Check sheet for the modelled part. Datum: model origin and axes. Units: mm. Face numbers are marked on the shaded views. A direction names the side the tool comes from. Coordinates: 2 decimals unless noted, no trailing zeros. Write each loop counter-clockwise with the first axis right and the second up, starting at its lowest first coordinate (ties: lowest second). Pieces come first, ordered by that corner, then holes. Notation, with made-up numbers: (-13, -35) -> (39, -35) arc R15 cw to (39, -14) -> close; hole circle Ø11 at (66.5, 21.5). An arc over 180 degrees is marked (long way). Put each result on its own line as item: value.
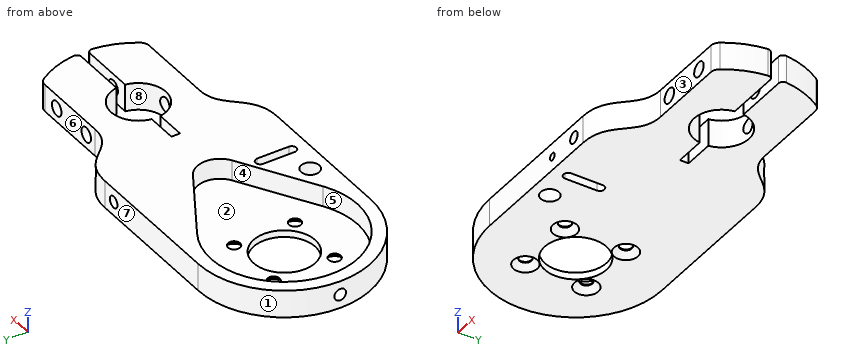
Autodesk Inventor part; units mm, degrees
ref_plane "Work Plane2" through (-108.2066, 0, 0) normal (1, 0, 0) x (0, 1, 0)
ref_plane "XZ Plane" through (0, 0, 0) normal (0, 1, 0) x (-1, 0, 0)
ref_plane "XY Plane" through (0, 0, 0) normal (0, 0, 1) x (1, 0, 0)
sketch "Sketch1" plane through (0, 0, 0) normal (0, 0, 1) x (1, 0, 0)
  circle A0 centre (-78.2066, 0) radius 10.75
  arc A1 (-78.2066, 30) -> (-78.2066, -30) centre (-78.2066, 0) ccw
  line L0 (-78.2066, 30) -> (-28.164, 30)
  line L1 (-28.164, -30) -> (-78.2066, -30)
  circle A2 centre (-88.8132, 10.6066) radius 2.1
  circle A3 centre (-67.6, -10.6066) radius 2.1
  circle A4 centre (-88.8132, -10.6066) radius 2.1
  circle A5 centre (-67.6, 10.6066) radius 2.1
  line L2 (-88.8132, 10.6066) -> (-67.6, -10.6066) construction
  line L3 (-67.6, 10.6066) -> (-88.8132, -10.6066) construction
  line L4 (-67.6, 10.6066) -> (-88.8132, 10.6066) construction
  line L5 (-67.6, 10.6066) -> (-67.6, -10.6066) construction
  line L6 (-135.9764, 0) -> (58.4124, 0)
  line L7 (9.4315, 1.5) -> (28.2442, 1.5)
  line L8 (28.2442, -1.5) -> (9.4315, -1.5)
  line L9 (-9.4315, 1.5) -> (-29.9625, 1.5)
  line L10 (-9.4315, -1.5) -> (-29.9625, -1.5)
  line L11 (-20, -1.5) -> (-20, 1.5)
  line L12 (9.55, -26.0565) -> (9.55, -21.3339)
  line L13 (12.725, -18.1589) -> (22.25, -18.1589)
  arc A6 (12.725, -18.1589) -> (9.55, -21.3339) centre (12.725, -21.3339) ccw
  arc A7 (7.1295, 29.1405) -> (0, 30) centre (0, 0) ccw
  arc A8 (9.4315, 1.5) -> (-9.4315, 1.5) centre (0, 0) ccw
  arc A9 (-9.4315, -1.5) -> (9.4315, -1.5) centre (0, 0) ccw
  arc A10 (24.8835, -16.7574) -> (29.8223, -3.26) centre (0, 0) ccw
  arc A11 (22.25, -18.1589) -> (24.8835, -16.7574) centre (22.25, -14.9839) ccw
  arc A12 (7.1295, -29.1405) -> (9.55, -26.0565) centre (6.375, -26.0565) ccw
  line L14 (9.55, 26.0565) -> (9.55, 21.3339)
  line L15 (12.725, 18.1589) -> (22.25, 18.1589)
  arc A13 (9.55, 21.3339) -> (12.725, 18.1589) centre (12.725, 21.3339) ccw
  arc A14 (29.8223, 3.26) -> (24.8835, 16.7574) centre (0, 0) ccw
  arc A15 (24.8835, 16.7574) -> (22.25, 18.1589) centre (22.25, 14.9839) ccw
  arc A16 (9.55, 26.0565) -> (7.1295, 29.1405) centre (6.375, 26.0565) ccw
  arc A17 (0, -30) -> (7.1295, -29.1405) centre (0, 0) ccw
  arc A18 (0, 30) -> (0, -30) centre (0, 0) ccw construction
  line L16 (-28.164, -30) -> (-14.7272, -30) construction
  line L17 (-14.7272, -30) -> (-16.1546, -18.1589) construction
  line L18 (-16.1546, -18.1589) -> (-4.7625, -18.1589) construction
  spline S0 degree 3 poles (-28.164, -30) (-14.7272, -30) (-16.1546, -18.1589) (-4.7625, -18.1589) knots 1 1 1 1 2 2 2 2
  arc A19 (28.2442, 1.5) -> (29.8223, 3.26) centre (28.2442, 3.0875) ccw
  arc A20 (29.8223, -3.26) -> (28.2442, -1.5) centre (28.2442, -3.0875) ccw
  line L19 (12.725, -18.1589) -> (-4.7625, -18.1589)
  line L20 (-28.164, 30) -> (-14.7272, 30) construction
  line L21 (-14.7272, 30) -> (-16.1546, 18.1589) construction
  line L22 (-16.1546, 18.1589) -> (-4.7625, 18.1589) construction
  spline S1 degree 3 poles (-28.164, 30) (-14.7272, 30) (-16.1546, 18.1589) (-4.7625, 18.1589) knots 1 1 1 1 2 2 2 2
  line L23 (12.725, 18.1589) -> (-4.7625, 18.1589)
  point P0 (-78.2066, 0)
  point P1 (9.55, -28.4394)
  point P2 (9.55, -18.1589)
  point P3 (23.88, -18.1589)
  point P4 (23.88, -18.1589)
  point P5 (29.9625, -1.5)
  point P6 (9.55, 28.4394)
  point P7 (9.55, 18.1589)
  point P8 (23.88, 18.1589)
  point P9 (23.88, 18.1589)
  point P10 (29.9625, 1.5)
  dimension "d2" = 21.5
  dimension "d3" = 78.2066
  dimension "d4" = 60
  dimension "d5" = 4.2
  dimension "d6" = 4.2
  dimension "d7" = 4.2
  dimension "d8" = 4.2
  dimension "d9" = 30
  dimension "d13" = 3
  dimension "d20" = 3
  dimension "d21" = 1.5
  dimension "d22" = 20
  dimension "d34" = 3.175
  dimension "d35" = 30
  dimension "d38" = 9.55
  dimension "d39" = 9.55
  dimension "d41" = 30
  dimension "d43" = 3.175
  dimension "d44" = 9.525
  dimension "d45" = 3.175
  dimension "d49" = 1.5875
  dimension "d85" = 4.7625
extrude "Extrusion4" add sketch "Sketch1" along normal blind 9.525 contours L6 L11 L10 A9 L8 A20 A10 A11 L13 L19 S0 L1 A1 A0 | A0 L6 A1 L0 S1 L23 L15 A15 A14 A19 L7 A8 L9 L11
sketch "Sketch4" plane through (0, 0, 9.525) normal (0, 0, 1) x (1, 0, 0)
  circle A0 centre (-78.2066, 0) radius 10.75
  arc A1 (-65.2016, 21.9344) -> (-65.2016, -21.9344) centre (-78.2066, 0) ccw
  line L0 (-65.2016, 21.9344) -> (-39.7222, 6.8276)
  line L1 (-39.7222, -6.8276) -> (-65.2016, -21.9344)
  line L2 (-135.8143, 0) -> (57.4394, 0)
  arc A2 (-39.7222, -6.8276) -> (-39.7222, 6.8276) centre (-43.7703, 0) ccw
  point P0 (0, 0)
  point P1 (-28.2066, 0)
  dimension "d28" = 51
  dimension "d29" = 50
  dimension "d30" = 7.9375
extrude "Extrusion6" cut sketch "Sketch4" against normal blind 7.1437 contours L2 A2 L1 A1 A0 | A0 L2 A1 L0 A2
sketch "Sketch5" plane through (12.675, 18.1589, 0) normal (0, 1, 0) x (1, 0, 0)
  line L0 (9.575, 0) -> (9.575, -9.525) construction
  line L1 (-3.2435, 0) -> (-3.2435, -9.525) construction
  line L2 (9.575, 0) -> (-17.4375, 0)
  line L3 (9.575, -9.525) -> (-17.4375, -9.525)
  line L4 (9.575, 0) -> (-3.2435, 0) construction
  line L5 (-3.2435, -9.525) -> (9.575, -9.525) construction
  circle A0 centre (3.1657, -4.7625) radius 2.5527
  line L6 (-22.1065, 0) -> (-22.1065, -9.525)
  line L7 (-22.1065, 0) -> (-3.2435, 0) construction
  circle A1 centre (-12.675, -4.7625) radius 2.5527
  point P0 (-3.2435, -4.7625)
  point P1 (3.1657, 0)
  point P2 (-12.675, 0)
  dimension "d86" = 5.1054
  dimension "d87" = 5.1054
extrude "Extrusion7" cut sketch "Sketch5" against normal through all
sketch "Sketch6" plane through (-78.2066, 30, 0) normal (0, 1, 0) x (1, 0, 0)
  line L0 (50.0426, 0) -> (0, 0)
  line L1 (0, 0) -> (0, -9.525)
  line L2 (50.0426, -9.525) -> (0, -9.525)
  line L3 (50.0426, 0) -> (50.0426, -9.525)
  circle A0 centre (45.2801, -4.7625) radius 2.0193
  point P0 (78.2066, 0)
  point P1 (50.0426, -4.7625)
  dimension "d50" = 4.0386
  dimension "d51" = 4.7625
extrude "Extrusion8" cut sketch "Sketch6" against normal blind 12.7 contours A0
thread "Thread2"
mirror "Mirror1" about plane through (0, 0, 0) normal (0, 1, 0) of "Extrusion8"
ref_plane "Work Plane2" through (-108.2066, 0, 0) normal (1, 0, 0) x (0, 1, 0)
sketch "Sketch7" plane through (-108.2066, 0, 0) normal (1, 0, 0) x (0, 1, 0)
  line L0 (30, 0) -> (-30, 0)
  line L1 (-30, 0) -> (-30, 9.525)
  line L2 (30, 9.525) -> (-30, 9.525)
  line L3 (30, 0) -> (30, 9.525)
  circle A0 centre (0, 4.7625) radius 2.0193
  point P0 (0, 0)
  point P1 (-30, 4.7625)
  point P2 (0, 9.525)
  dimension "d54" = 4.0386
extrude "Extrusion9" cut sketch "Sketch7" along normal up to surface contours A0
sketch "Sketch8" plane through (0, 0, 9.525) normal (0, 0, 1) x (1, 0, 0)
  circle A0 centre (-67.6, 10.6066) radius 2.1
  circle A1 centre (-88.8132, -10.6066) radius 2.1
  circle A2 centre (-67.6, -10.6066) radius 2.1
  circle A3 centre (-88.8132, 10.6066) radius 2.1
  circle A4 centre (-78.2066, 0) radius 10.75
  arc A5 (-65.2016, 21.9344) -> (-65.2016, -21.9344) centre (-78.2066, 0) ccw
  line L0 (-39.7222, -6.8276) -> (-65.2016, -21.9344)
  arc A6 (-39.7222, -6.8276) -> (-39.7222, 6.8276) centre (-43.7703, 0) ccw
  line L1 (-65.2016, 21.9344) -> (-39.7222, 6.8276)
  line L2 (-39.7222, -6.8276) -> (-65.2016, -21.9344)
  arc A7 (-65.2016, 21.9344) -> (-65.2016, -21.9344) centre (-78.2066, 0) ccw
  line L3 (-65.2016, 21.9344) -> (-39.7222, 6.8276)
  arc A8 (-39.7222, -6.8276) -> (-39.7222, 6.8276) centre (-43.7703, 0) ccw
  arc A9 (-78.2066, 30) -> (-78.2066, -30) centre (-78.2066, 0) ccw
  line L4 (-78.2066, -30) -> (-28.164, -30)
  line L5 (-4.7625, -18.1589) -> (22.25, -18.1589)
  arc A10 (22.25, -18.1589) -> (24.8835, -16.7574) centre (22.25, -14.9839) ccw
  arc A11 (24.8835, -16.7574) -> (29.8223, -3.26) centre (0, 0) ccw
  arc A12 (29.8223, -3.26) -> (28.2442, -1.5) centre (28.2442, -3.0875) ccw
  line L6 (28.2442, -1.5) -> (9.4315, -1.5)
  arc A13 (-9.4315, -1.5) -> (9.4315, -1.5) centre (0, 0) ccw
  line L7 (-9.4315, -1.5) -> (-20, -1.5)
  line L8 (-20, -1.5) -> (-20, 1.5)
  line L9 (-20, 1.5) -> (-9.4315, 1.5)
  arc A14 (9.4315, 1.5) -> (-9.4315, 1.5) centre (0, 0) ccw
  line L10 (9.4315, 1.5) -> (28.2442, 1.5)
  arc A15 (28.2442, 1.5) -> (29.8223, 3.26) centre (28.2442, 3.0875) ccw
  arc A16 (29.8223, 3.26) -> (24.8835, 16.7574) centre (0, 0) ccw
  arc A17 (24.8835, 16.7574) -> (22.25, 18.1589) centre (22.25, 14.9839) ccw
  line L11 (22.25, 18.1589) -> (-4.7625, 18.1589)
  line L12 (-28.164, 30) -> (-78.2066, 30)
  circle A18 centre (-55.6441, -23.65) radius 3.175
  line L13 (-135.9764, 0) -> (58.4124, 0)
  dimension "d57" = 6.35
  dimension "d58" = 6.35
  dimension "d59" = 6.35
extrude "Extrusion10" cut sketch "Sketch8" against normal through all contours A18
chamfer "Chamfer1" distance 2.05 angle 45 4 edges at (-69.7, -10.6066, 0) (-69.7, 10.6066, 0) (-90.9132, 10.6066, 0) (-90.9132, -10.6066, 0) measured on face at (-37.888, 14.0355, 0)
sketch "Sketch9" plane through (0, 0, 0) normal (0, 0, -1) x (-1, 0, 0)
  circle A0 centre (78.2066, 0) radius 10.75
  arc A1 (-9.4315, -1.5) -> (9.4315, -1.5) centre (0, 0) ccw
  arc A2 (9.4315, 1.5) -> (-9.4315, 1.5) centre (0, 0) ccw
  arc A3 (80.5159, -8.2842) -> (80.5159, 8.2842) centre (78.2066, 0) ccw
  arc A4 (7.9482, 28.5129) -> (7.9482, -28.5129) centre (0, 0) ccw
  line L0 (7.9482, 28.5129) -> (80.5159, 8.2842)
  line L1 (80.5159, -8.2842) -> (7.9482, -28.5129)
  circle A5 centre (55.6441, -23.65) radius 3.175
  line L2 (34.9458, -30) -> (30.9072, -30)
  circle A6 centre (55.6441, -23.65) radius 3.175
  line L3 (52.4691, -23.65) -> (52.4691, -30) construction
  line L4 (52.4691, -30) -> (34.9458, -30)
  circle A7 centre (44.5012, -22.476) radius 4 construction
  arc A8 (42.9012, -24.476) -> (46.1012, -24.476) centre (44.5012, -24.476) ccw
  arc A9 (46.1012, -13.476) -> (42.9012, -13.476) centre (44.5012, -13.476) ccw
  line L5 (46.1012, -24.476) -> (46.1012, -13.476)
  line L6 (42.9012, -13.476) -> (42.9012, -24.476)
  point P0 (43.7074, -30)
  dimension "d65" = 17.2
  dimension "d66" = 59.2
  dimension "d67" = 8
  dimension "d68" = 3.2
  dimension "d69" = 3.2
  dimension "d70" = 2
  dimension "d71" = 11
  dimension "d84" = 0.7937
extrude "Extrusion11" cut sketch "Sketch9" against normal through all contours L5 A8 L6 L1 | L1 L6 A9 L5
sketch "Sketch10" plane through (-78.2066, -30, 0) normal (0, -1, 0) x (1, 0, 0)
  line L0 (35.3054, 0) -> (35.3054, 9.525)
  line L1 (32.1054, 0) -> (32.1054, 9.525)
  circle A0 centre (33.7054, 4.7625) radius 1.25
  line L2 (35.3054, 9.525) -> (32.1054, 9.525) construction
  point P0 (78.2066, 0)
  point P1 (32.1054, 4.7625)
  point P2 (33.7054, 9.525)
  dimension "d74" = 2.5
extrude "Extrusion12" cut sketch "Sketch10" against normal up to surface
thread "Thread1"
thread "Thread3"
equation "\"d4\" = mount_diameter"
equation "\"d9\" = hole_pattern_diameter"
equation "\"d13\" = clamp_slit"
equation "\"d20\" = clamp_slit"
equation "\"d21\" = 0.5 * clamp_slit"
equation "\"d35\" = 0.5 * mount_diameter"
equation "\"d41\" = 0.5 * mount_diameter"
equation "\"d23\" = thickness"
equation "\"d31\" = thickness - motor_mount_thickness"
equation "\"mount_diameter\" = 60"
equation "\"center_distance\" = 78.2066"
equation "\"hole_pattern_diameter\" = 30"
equation "\"thickness\" = 9.525"
equation "\"clamp_slit\" = 3"
equation "\"motor_mount_thickness\" = 2.38125"
properties part number "MotorMount" material "Aluminum 6061"
Q1. Tool access check on the marked faces 5, 6, 7 and 8. Record the directions out of +Z, -Z, +X, -X, +Y, -Y that give a thin tool (end or side, any length) a straight path to the whole face; none if there is none.
Recorded:
face 5: +Z
face 6: +Z, -Z, +X, +Y
face 7: +Z, -Z, +X, -X, +Y
face 8: +Z, -Z
Q2. Cross-section at A-A (y = 0). Record the cut outline in (x, z) (3 decimals), plus the area to 3 significant figures.
Recorded:
outline: (-108.207, 0) -> (-88.957, 0) -> (-88.957, 2.381) -> (-103.707, 2.381) -> (-103.707, 2.743) -> (-108.207, 2.743) -> close; (-108.207, 6.782) -> (-103.707, 6.782) -> (-103.707, 9.525) -> (-108.207, 9.525) -> close; (-67.457, 0) -> (-20, 0) -> (-20, 9.525) -> (-35.833, 9.525) -> (-35.833, 2.381) -> (-67.457, 2.381) -> close
area: 286 mm2
Q3. Depth check by flat-ended pin: P1, Ø4.5, axis at y = 0, z = 4.76, coming from the +X side; P2, Ø4, axis at x = -55.64, y = -23.65, coming from the +Z side; P3, Ø24.5, axis at x = -78.21, y = 0, coming from the +Z side; P4, Ø3, axis at x = 1, z = 2, coming from the +Y side. Enter the tip coordinate at first touch or a pass-through.
Recorded:
P1: stops at x = 29.59
P2: passes through
P3: stops at z = 2.38
P4: stops at y = 18.16
Q4. Mould release check, pull along X, two halves, no side actions. Record for the marked faces 1, 2, 3 and 4: released by +X, released by -X, zero draft, split by the parting line, or undercut.
Recorded:
face 1: released by -X
face 2: undercut
face 3: zero draft
face 4: undercut
Q5. Cross-section at B-B (x = -54). Record the cut outline in (y, z) (3 decimals), plus the area to 3 significant figures.
Recorded:
outline: (-30, 0) -> (-26.366, 0) -> (-26.366, 9.525) -> (-30, 9.525) -> close; (-20.934, 0) -> (30, 0) -> (30, 9.525) -> (15.293, 9.525) -> (15.293, 2.381) -> (-15.293, 2.381) -> (-15.293, 9.525) -> (-20.934, 9.525) -> close
area: 301 mm2
Q6. Material ranges on line 1 along Y through (x, z) = (11.5, 7.5); line 2 along X through (y, z) = (-3, 7.5); line 3 along X through (y, z) = (-2, 9), recorded low to high.
Recorded:
line 1: y = -18.16 to -1.5, 1.5 to 18.16
line 2: x = -108.06 to -103.53, -36.42 to -9.07, 9.07 to 29.83
line 3: x = -108.14 to -103.63, -36.09 to -9.34, 9.34 to 29.4
Q7. Cross-section at C-C (x = 1). Record the cut outline in (y, z) (3 decimals).
Recorded:
outline: (-18.159, 0) -> (-9.498, 0) -> (-9.498, 2.414) -> (-18.159, 2.414) -> close; (-18.159, 7.111) -> (-9.498, 7.111) -> (-9.498, 9.525) -> (-18.159, 9.525) -> close; (9.498, 0) -> (18.159, 0) -> (18.159, 2.414) -> (9.498, 2.414) -> close; (9.498, 7.111) -> (18.159, 7.111) -> (18.159, 9.525) -> (9.498, 9.525) -> close
Q8. Cross-section at D-D (x = 15). Record the cut outline in (y, z) (3 decimals), plus the area to 3 significant figures.
Recorded:
outline: (-18.159, 0) -> (-1.5, 0) -> (-1.5, 2.352) -> (-18.159, 2.352) -> close; (-18.159, 7.173) -> (-1.5, 7.173) -> (-1.5, 9.525) -> (-18.159, 9.525) -> close; (1.5, 0) -> (18.159, 0) -> (18.159, 2.352) -> (1.5, 2.352) -> close; (1.5, 7.173) -> (18.159, 7.173) -> (18.159, 9.525) -> (1.5, 9.525) -> close
area: 157 mm2
